Check sheet for the modelled part. Datum: model origin and axes. Units: mm. A direction names the side the tool comes from. Round coordinates to 2 decimals unless told otherwise and drop trailing zeros. Loops run counter-clockwise (first coordinate to the right, second up) from the corner with the lowest first, then second, coordinate; pieces in that order, holes last. Notation, with made-up numbers: M 69.5,-15.75 L 90.5,-15.75 A14 ccw 90.5,6.25 Z; hole C 58.5,17.5 d3. An arc over 180 degrees is marked long. Write item = value, one per line. Start each with the question number.
(1) Cross-section at A-A on z = 7.5. Record the boundary of the cut face in (x, y) (3 decimals), plus the area to 3 significant figures.
(2) Go/stop test with a flat-tipped pin: P1, Ø5, axis at y = 3, z = 8, coming from the +X side (3 decimals). Record where the tip stops, or that it passes through.
(3) Cross-section at B-B on x = -23.6. Record the boundary of the cut face in (y, z) (3 decimals).
(4) Scan lines: L1, parallel to Y at x = -24.55, z = 2.5 (3 decimals); L2, parallel to X at y = 17, z = 11 (3 decimals); L3, parallel to Z at x = -22.55, y = 4.5. Record each from-to range of solid material in increasing order. Write a range as from..to.
(5) Set-up check for faces 1 (the face through (-26, -19.375, 3)), 2 (the face through (-24, 18.625, 7)): record each of +Z, -Z, +X, -X, +Y, -Y from which the full face is reachable in a straight line by a thin tool's end or side.
from build123d import *

# Parameters (mm, degrees)
SKETCH1_W           = 4.25
SKETCH1_H           = 38.75
BOSS_EXTRUDE1_DEPTH = 12
SKETCH2_W           = 9.75
SKETCH2_H           = 38
CUT_EXTRUDE1_DEPTH  = 3.5


with BuildPart() as part:
    # Sketch1 → Boss-Extrude1 (new body)
    with BuildSketch(Plane.XY):
        Rectangle(SKETCH1_W, SKETCH1_H)
    extrude(amount=BOSS_EXTRUDE1_DEPTH)

    # Sketch2 → Cut-Extrude1 (cut)
    with BuildSketch(Plane.ZY.offset(2.125)):
        with Locations((7.125, -0.375)):
            Rectangle(SKETCH2_W, SKETCH2_H)
    extrude(amount=-CUT_EXTRUDE1_DEPTH, mode=Mode.SUBTRACT)


with BuildPart() as body_2:
    # Mirror2: mirrored copy
    add(part.part.mirror(Plane.ZY.offset(12.125)))


solid = body_2.part
Result:
q1.outline = M -26.375,-19.375 L -25.625,-19.375 L -25.625,18.625 L -22.125,18.625 L -22.125,19.375 L -26.375,19.375 Z
q1.area = 31.7 mm^2
q2.P1 = -25.625
q3.outline = M -19.375,0 L 19.375,0 L 19.375,12 L 18.625,12 L 18.625,2.25 L -19.375,2.25 Z
q4.L1 = 18.625..19.375
q4.L2 = -26.375..-25.625
q4.L3 = 0..2.25
q5.face_1 = +Z, -Z, +X, -X, -Y
q5.face_2 = +Z, +X, -Y
